Read the model definition and answer for the solid it produces. Units are mm, in the model's axes. A direction names the side the tool comes from. Round coordinates to 2 decimals unless told otherwise and drop trailing zeros. Write each loop counter-clockwise with the first axis right and the second up, starting at its lowest first coordinate (ties: lowest second). Pieces come first, ordered by that corner, then holes. Notation, with made-up numbers: (55.25, 56.5) -> (103.25, 56.5) arc R17 cw to (103.25, 88.5) -> close; hole circle Ø7 at (50.25, 82.5). An arc over 180 degrees is marked (long way). Return JSON: item names as keys, results as strings.
from build123d import *

# Parameters (mm, degrees)
SKETCH1_W           = 122
SKETCH1_H           = 18
SKETCH1_R           = 1.3
BOSS_EXTRUDE1_DEPTH = 8
CUT_EXTRUDE1_DEPTH  = 3
SKETCH3_W           = 10
SKETCH3_H           = 4
CUT_EXTRUDE2_DEPTH  = 4
SKETCH4_R           = 1.3
CUT_EXTRUDE3_DEPTH  = 10
SKETCH5_W           = 2
SKETCH5_H           = 5
CUT_EXTRUDE4_DEPTH  = 10


with BuildPart() as part:
    # Sketch1 → Boss-Extrude1 (new body)
    with BuildSketch(Plane.XY):
        Rectangle(SKETCH1_W, SKETCH1_H)
        with Locations((-26, 5)):
            Circle(SKETCH1_R, mode=Mode.SUBTRACT)
        with Locations((-36, 5)):
            Circle(SKETCH1_R, mode=Mode.SUBTRACT)
        with Locations((-26, -5)):
            Circle(SKETCH1_R, mode=Mode.SUBTRACT)
        with Locations((-36, -5)):
            Circle(SKETCH1_R, mode=Mode.SUBTRACT)
        with Locations((26, -5)):
            Circle(SKETCH1_R, mode=Mode.SUBTRACT)
        with Locations((36, -5)):
            Circle(SKETCH1_R, mode=Mode.SUBTRACT)
        with Locations((36, 5)):
            Circle(SKETCH1_R, mode=Mode.SUBTRACT)
        with Locations((26, 5)):
            Circle(SKETCH1_R, mode=Mode.SUBTRACT)
    extrude(amount=BOSS_EXTRUDE1_DEPTH)

    # Sketch2 → Cut-Extrude1 (cut)
    with BuildSketch(Plane(origin=(0, 0, 0), x_dir=(-1, 0, 0), z_dir=(0, 0, -1))):
        Polygon((-36, 2), (-33.401923789, 3.5), (-33.401923789, 6.5), (-36, 8), (-38.598076211, 6.5), (-38.598076211, 3.5), align=None)
        Polygon((-26, 2), (-23.401923789, 3.5), (-23.401923789, 6.5), (-26, 8), (-28.598076211, 6.5), (-28.598076211, 3.5), align=None)
        Polygon((-26, -8), (-23.401923789, -6.5), (-23.401923789, -3.5), (-26, -2), (-28.598076211, -3.5), (-28.598076211, -6.5), align=None)
        Polygon((-36, -8), (-33.401923789, -6.5), (-33.401923789, -3.5), (-36, -2), (-38.598076211, -3.5), (-38.598076211, -6.5), align=None)
        Polygon((26, 2), (28.598076211, 3.5), (28.598076211, 6.5), (26, 8), (23.401923789, 6.5), (23.401923789, 3.5), align=None)
        Polygon((26, -8), (28.598076211, -6.5), (28.598076211, -3.5), (26, -2), (23.401923789, -3.5), (23.401923789, -6.5), align=None)
        Polygon((36, -8), (38.598076211, -6.5), (38.598076211, -3.5), (36, -2), (33.401923789, -3.5), (33.401923789, -6.5), align=None)
        Polygon((36, 2), (38.598076211, 3.5), (38.598076211, 6.5), (36, 8), (33.401923789, 6.5), (33.401923789, 3.5), align=None)
    extrude(amount=-CUT_EXTRUDE1_DEPTH, mode=Mode.SUBTRACT)

    # Sketch3 → Cut-Extrude2 (cut)
    with BuildSketch(Plane(origin=(0, 0, 0), x_dir=(-1, 0, 0), z_dir=(0, 0, -1))):
        with Locations((-56, 7)):
            Rectangle(SKETCH3_W, SKETCH3_H)
        with Locations((56, 7)):
            Rectangle(SKETCH3_W, SKETCH3_H)
    extrude(amount=-CUT_EXTRUDE2_DEPTH, mode=Mode.SUBTRACT)

    # Sketch4 → Cut-Extrude3 (cut)
    with BuildSketch(Plane(origin=(61, 0, 0), x_dir=(0, 0, -1), z_dir=(1, 0, 0))):
        with Locations((-4, 0)):
            Circle(SKETCH4_R)
    cut_extrude3 = extrude(amount=-CUT_EXTRUDE3_DEPTH, mode=Mode.SUBTRACT)

    # Sketch5 → Cut-Extrude4 (cut)
    with BuildSketch(Plane(origin=(0, 0, 0), x_dir=(-1, 0, 0), z_dir=(0, 0, -1))):
        with Locations((-52, 0)):
            Rectangle(SKETCH5_W, SKETCH5_H)
    cut_extrude4 = extrude(amount=-CUT_EXTRUDE4_DEPTH, mode=Mode.SUBTRACT)

    # Mirror1: Cut-Extrude3, Cut-Extrude4 across plane
    add(cut_extrude3.mirror(Plane(origin=(0, 0, 0), x_dir=(0, 0, 1), z_dir=(1, 0, 0))), mode=Mode.SUBTRACT)
    add(cut_extrude4.mirror(Plane(origin=(0, 0, 0), x_dir=(0, 0, 1), z_dir=(1, 0, 0))), mode=Mode.SUBTRACT)


solid = part.part
Item 1: Straight lines are drawn through the part: L1, parallel to X at y = -5.75, z = 0.75; L2, parallel to X at y = 0.75, z = 5.5; L3, parallel to X at y = 5, z = 5.55. For each, find the intervals that lie inside material, in ascending order. Write a range as [from, to].
Worked answers:
{"L1": "x = [-61, -38.6], [-33.4, -28.6], [-23.4, 23.4], [28.6, 33.4], [38.6, 61]", "L2": "x = [-61, -53], [-51, 51], [53, 61]", "L3": "x = [-61, -37.3], [-34.7, -27.3], [-24.7, 24.7], [27.3, 34.7], [37.3, 61]"}
Item 2: Section B-B (y = -5) is taken. State how many separate pieces and enclosed holes the cut face has, then the cut area to 3 significant figures.
Worked answers:
{"separate pieces": "5", "enclosed holes": "0", "area": "862 mm2"}
Item 3: For a pull along X with two mould halves and no side action, classify faces 1 (the flat face through (27.28, 7.26, 1.48)), 2 (the flat face through (-1, -9, 4)) as released by +X, released by -X, zero draft, split by the parting line, or undercut.
Worked answers:
{"face 1": "undercut", "face 2": "zero draft"}
Item 4: Section A-A (x = -52) is taken. Give the vertices of the cut face in (y, z).
Worked answers:
{"outline": "(-9, 0) -> (-2.5, 0) -> (-2.5, 8) -> (-9, 8) -> close; (2.5, 0) -> (5, 0) -> (5, 4) -> (9, 4) -> (9, 8) -> (2.5, 8) -> close"}
Item 5: A tool of negligible diameter and unlimited length cuts with its end or side. For faces 3 (the flat face through (-1, 0, 8)), 4 (the flat face through (-53, -1.15, 3.06)), 5 (the flat face through (-27.32, -2.76, 1.48)), from which of +Z, -Z, +X, -X, +Y, -Y can it reach the whole face along a straight path? Write none if from no direction.
Worked answers:
{"face 3": "+Z, +X, -X, +Y, -Y", "face 4": "+Z, -Z", "face 5": "-Z"}
Item 6: A flat-ended cylindrical pin translates along its axis: pin 1 (2 mm diameter, centred on x = 36, y = -5, fed in from +Z). Find the tip coordinate at first contact, or state that the pin passes through.
Worked answers:
{"pin 1": "passes through"}
